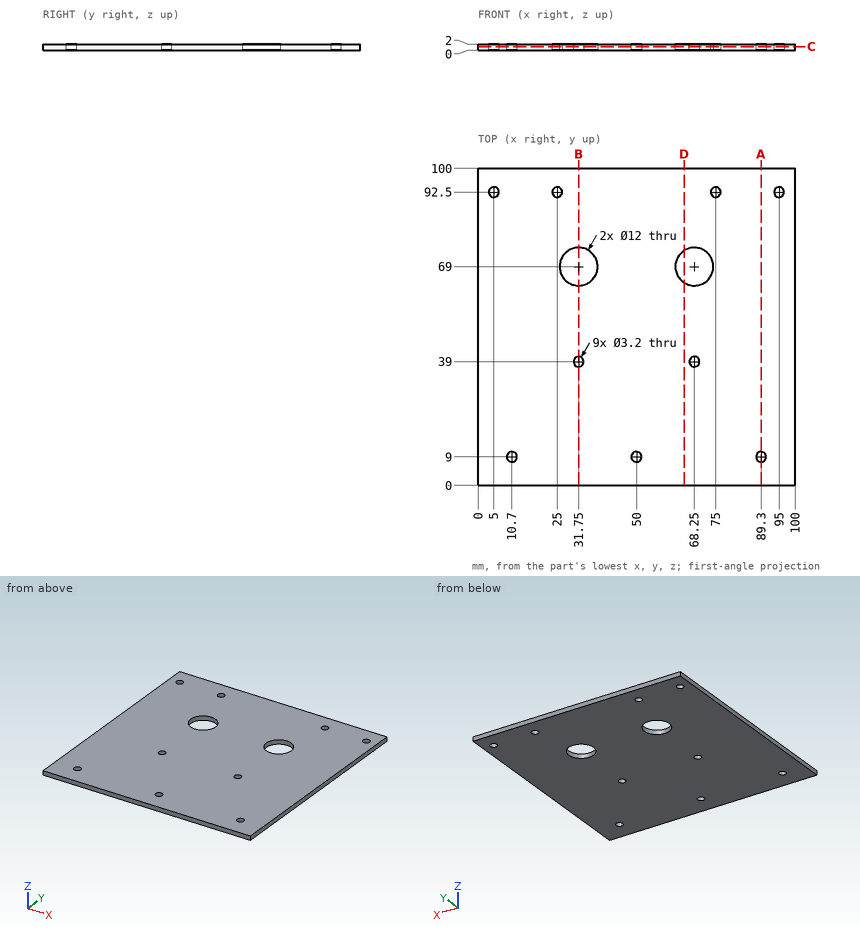
Verification items for this drawing (mm, ordinates from the low corner). Coordinates: 2 decimals unless noted, no trailing zeros. Loops run counter-clockwise (first coordinate to the right, second up) from the corner with the lowest first, then second, coordinate; pieces in that order, holes last. Notation, with made-up numbers: (-10, 49.5) -> (18, 49.5) arc R28 ccw to (18, 87.5) -> close; hole circle Ø3 at (38, 59.5). An arc over 180 degrees is marked (long way). Put each result on its own line as item: value.
1. Section check A-A, the plane x = 89.3. Record the boundary of the cut face in (y, z), then the cut area to 3 significant figures.
Result set:
outline: (0, 0) -> (7.4, 0) -> (7.4, 2) -> (0, 2) -> close; (10.6, 0) -> (100, 0) -> (100, 2) -> (10.6, 2) -> close
area: 194 mm^2
2. Section check D-D, the plane x = 65. Record the boundary of the cut face in (y, z), then the cut area to 3 significant figures.
Result set:
outline: (0, 0) -> (63.96, 0) -> (63.96, 2) -> (0, 2) -> close; (74.04, 0) -> (100, 0) -> (100, 2) -> (74.04, 2) -> close
area: 180 mm^2
3. Thickness scan on line 1 (Y direction, x = 68.5, z = 1.45); line 2 (X direction, y = 92.5, z = 0.5); line 3 (Y direction, x = 95, z = 1.35). Record the ranges inside material, lowest first.
Result set:
line 1: y = 0 to 37.42, 40.58 to 63.01, 74.99 to 100
line 2: x = 0 to 3.4, 6.6 to 23.4, 26.6 to 73.4, 76.6 to 93.4, 96.6 to 100
line 3: y = 0 to 90.9, 94.1 to 100
4. Section check B-B, the plane x = 31.75. Record the boundary of the cut face in (y, z).
Result set:
outline: (0, 0) -> (37.4, 0) -> (37.4, 2) -> (0, 2) -> close; (40.6, 0) -> (63, 0) -> (63, 2) -> (40.6, 2) -> close; (75, 0) -> (100, 0) -> (100, 2) -> (75, 2) -> close
5. Section check C-C, the plane z = 1.15. Give the number of separate pieces and of enclosed holes in the cut face, then the cut area to 3 significant figures.
Result set:
separate pieces: 1
enclosed holes: 11
area: 9,700 mm^2
6. Gauge pin test, flat ends, axial feed: P1, Ø2.5, axis at x = 95, y = 92.5, coming from the -Z side; P2, Ø4, axis at x = 89.3, y = 9, coming from the +Z side. Record the tip position at first contact, or that the pin passes through.
Result set:
P1: passes through
P2: stops at z = 2
